Can you work these out from the drawing? Everything is in mm from the part's minimum corner. A direction names the side the tool comes from. Round coordinates to 2 decimals unless told otherwise and drop trailing zeros. Order: outer loops, then holes, each group sorted by start corner. A loop starts at its lowest first (then second) coordinate and runs counter-clockwise, first axis right, second up. Notation, with made-up numbers: (23.5, 24.25) -> (46.5, 24.25) arc R17 cw to (46.5, 56.25) -> close; hole circle Ø9 at (54, -33.5). An arc over 180 degrees is marked (long way). Use a Markdown table: item, result. Add a question column.
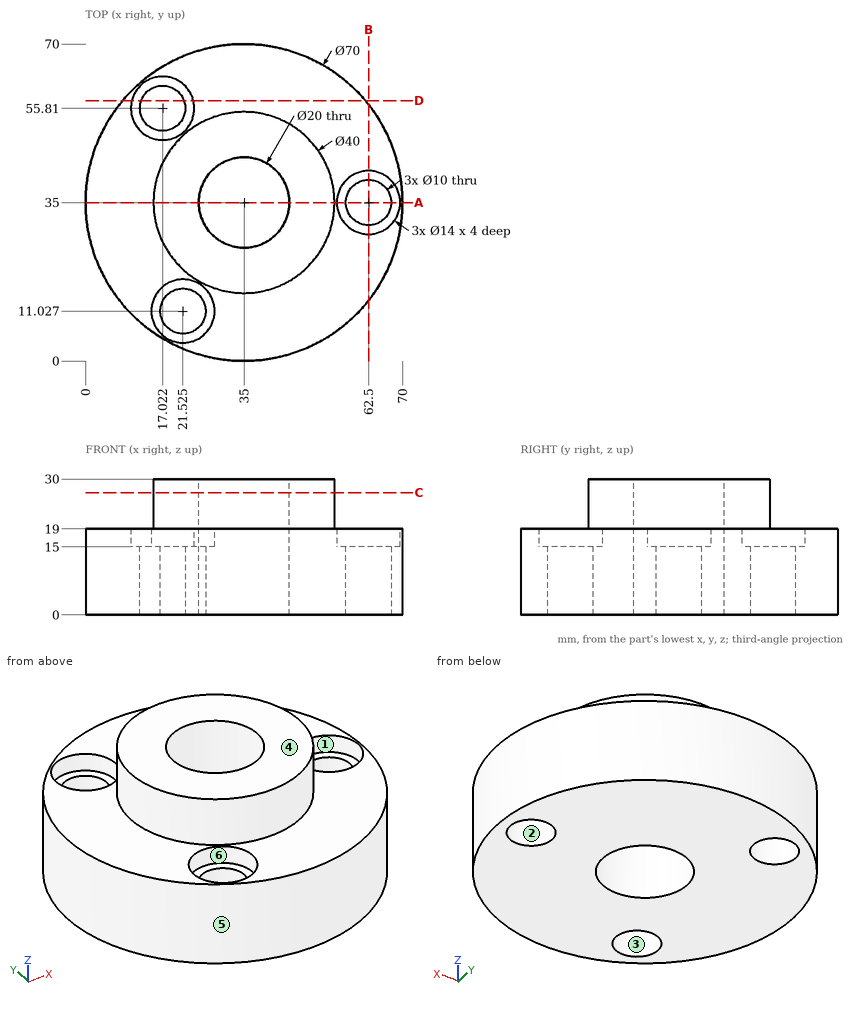
(1) I want a section at C-C on z = 27. List the corners of the cut face in (x, y) for me.
(2) If we mould it in two halves opening along Y, with no side actions, what happens to the marked faces 3, 4, 5 and 6? For each: pulls with the +Y half, pulls with the -Y half, needs draft (parallel to the pull), parting line crosses it, or undercut.
(3) Please list where these lines run through material, in increasing order: probe 1 along Z at (x, y) = (60, 12.5); probe 2 along Y at (x, z) = (62.5, 5.75); probe 3 along Y at (x, z) = (65.5, 9) (1 decimal). Write a range as from..to.
(4) I want a section at D-D on y = 57.5. List the corners of the cut face in (x, z) for me (1 decimal), and give its area (3 significant figures).
(5) On a 3-axis mill with a long thin cutter (end or side, diameter ignored), from which of +Z, -Z, +X, -X, +Y, -Y can I reach the whole of each face in a straight line? I mean the marked faces 1 and 2. Say none if no direction works.
(6) I want a section at A-A on y = 35. List the corners of the cut face in (x, z) for me.
(7) I want a section at B-B on x = 62.5. List the corners of the cut face in (y, z) for me, and give its area (3 significant figures).
(8) I'm going to push flat-ended pins straight in: P1, Ø4, axis at x = 22, y = 8, coming from the +Z side; P2, Ø5, axis at x = 33.5, z = 13, coming from the -Y side; P3, Ø3, axis at x = 53, z = 5.5, coming from the +Y side; P4, Ø22.5, axis at x = 62.5, y = 35, coming from the -Z side. Where does each tip first touch, or does it pass through?
Output:
| question | item | result |
|---|---|---|
| 1 | outline | circle Ø40 at (35, 35); hole circle Ø20 at (35, 35) |
| 2 | face 3 | undercut |
| 2 | face 4 | needs draft |
| 2 | face 5 | parting line crosses it |
| 2 | face 6 | undercut |
| 3 | probe 1 | 0..19 |
| 3 | probe 2 | 13.35..30, 40..56.65 |
| 3 | probe 3 | 17.8..31, 39..52.2 |
| 4 | outline | (8.2, 0) -> (12.3, 0) -> (12.3, 15) -> (10.2, 15) -> (10.2, 19) -> (8.2, 19) -> close; (21.7, 0) -> (61.8, 0) -> (61.8, 19) -> (23.8, 19) -> (23.8, 15) -> (21.7, 15) -> close |
| 4 | area | 823 mm² |
| 5 | face 1 | +Z |
| 5 | face 2 | +Z, -Z |
| 6 | outline | (0, 0) -> (25, 0) -> (25, 30) -> (15, 30) -> (15, 19) -> (0, 19) -> close; (45, 0) -> (57.5, 0) -> (57.5, 15) -> (55.5, 15) -> (55.5, 19) -> (55, 19) -> (55, 30) -> (45, 30) -> close; (67.5, 0) -> (70, 0) -> (70, 19) -> (69.5, 19) -> (69.5, 15) -> (67.5, 15) -> close |
| 7 | outline | (13.35, 0) -> (30, 0) -> (30, 15) -> (28, 15) -> (28, 19) -> (13.35, 19) -> close; (40, 0) -> (56.65, 0) -> (56.65, 19) -> (42, 19) -> (42, 15) -> (40, 15) -> close |
| 7 | area | 617 mm² |
| 8 | P1 | z = 15 |
| 8 | P2 | y = 0 |
| 8 | P3 | y = 65.87 |
| 8 | P4 | z = 0 |
